Job drawing, mm, ordinate dimensions from the low corner. One solid piece. A direction names the side the tool comes from. Give positions to 0.01 mm unless a question says otherwise; leave off trailing zeros. Order: outer loops, then holes, each group sorted by start corner. A loop starts at its lowest first (then second) coordinate and runs counter-clockwise, first axis right, second up. Notation, with made-up numbers: (64, 3.25) - (120, 3.25) arc R26 ccw to (120, 17.25) - close; hole circle Ø1 at (71.25, 34.25). An arc over 180 degrees is marked (long way). Use a Markdown table: item, result. Add a question column.
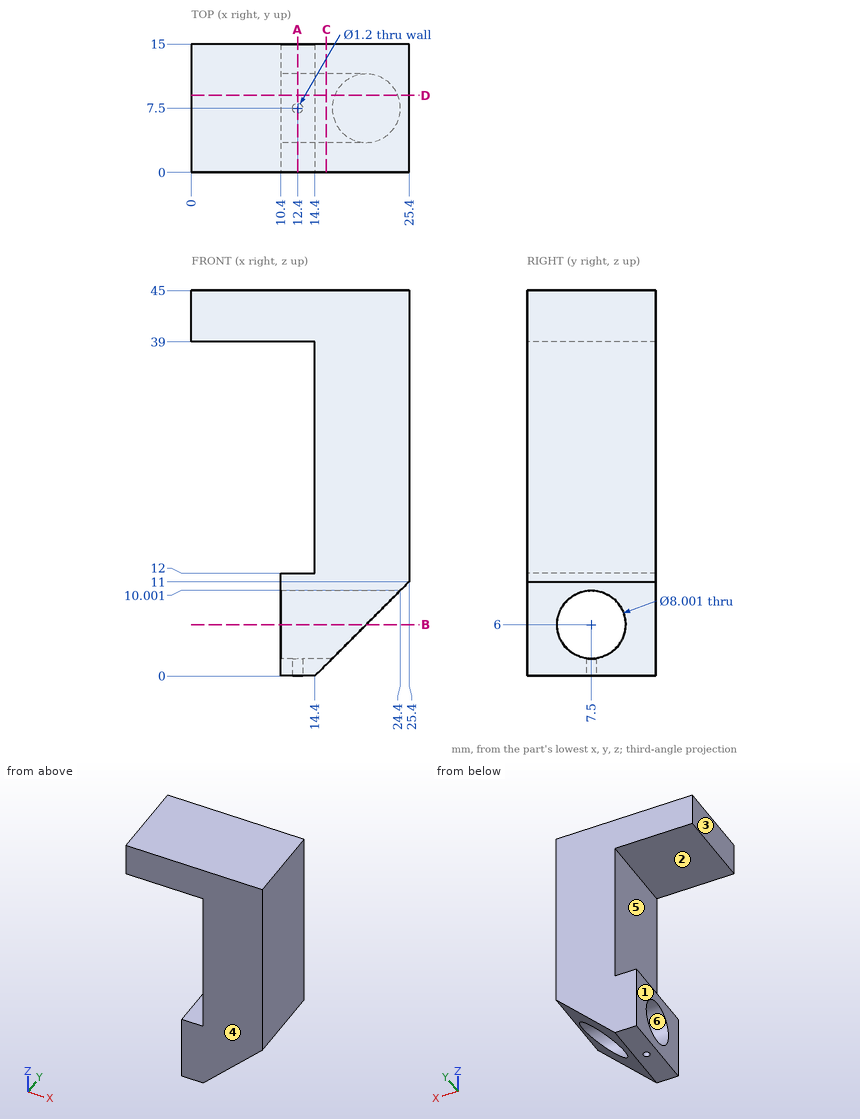
1. Mould opens along Y. For the marked faces 4, 5 and 6 say: released by +Y, released by -Y, zero draft, split by the parting line, or undercut.
2. Pin check, flat tips, straight feed: P1, Ø4.5, axis at y = 8, z = 29.5, coming from the -X side; P2, Ø9, axis at y = 7.5, z = 6, coming from the +X side; P3, Ø6, axis at x = 17.5, y = 7, coming from the -Z side. Stop position of each tip, or through.
3. Cut at B-B (z = 6). Write the cut outline in (x, y).
4. Cut at C-C (x = 15.75). Write the cut outline in (y, z).
5. Cut at A-A (x = 12.4). Write the cut outline in (y, z) (1 decimal), plus the area to 3 significant figures.
6. Cut at D-D (y = 9). Write the cut outline in (x, z), plus the area to 3 significant figures.
7. Drill centre lines: probe 1 along Y at (x, z) = (12.4, 0.9); probe 2 along Y at (x, z) = (14, 6); probe 3 along Z at (x, y) = (13.5, 7.5). Where is each one in solid material? Low to high. Write a range as [from, to].
8. Tool access for the marked faces 1, 2 and 3: list every direction of +Z, -Z, +X, -X, +Y, -Y with a clear straight run to the whole face (end or side of a thin tool).
Responses:
| question | item | result |
|---|---|---|
| 1 | face 4 | released by -Y |
| 1 | face 5 | zero draft |
| 1 | face 6 | undercut |
| 2 | P1 | stops at x = 14.4 |
| 2 | P2 | stops at x = 24.9 |
| 2 | P3 | stops at z = 0.1 |
| 3 | outline | (10.4, 0) - (20.4, 0) - (20.4, 3.5) - (10.4, 3.5) - close; (10.4, 11.5) - (20.4, 11.5) - (20.4, 15) - (10.4, 15) - close |
| 4 | outline | (0, 1.35) - (15, 1.35) - (15, 45) - (0, 45) - close; hole circle Ø8 at (7.5, 6) |
| 5 | outline | (0, 0) - (6.9, 0) - (6.9, 2) arc R4 cw (long way) to (8.1, 2) - (8.1, 0) - (15, 0) - (15, 12) - (0, 12) - close; (0, 39) - (15, 39) - (15, 45) - (0, 45) - close |
| 5 | area | 217 mm² |
| 6 | outline | (0, 39) - (14.4, 39) - (14.4, 12) - (10.4, 12) - (10.4, 9.71) - (24.11, 9.71) - (25.4, 11) - (25.4, 45) - (0, 45) - close; (10.4, 0) - (14.4, 0) - (16.69, 2.29) - (10.4, 2.29) - close |
| 6 | area | 495 mm² |
| 7 | probe 1 | y = [0, 6.9], [8.1, 15] |
| 7 | probe 2 | y = [0, 3.5], [11.5, 15] |
| 7 | probe 3 | z = [0, 2], [10, 12], [39, 45] |
| 8 | face 1 | -Z, -X, +Y, -Y |
| 8 | face 2 | -X, +Y, -Y |
| 8 | face 3 | +Z, -Z, -X, +Y, -Y |
